```python
from build123d import *

# Parameters (mm, degrees)
SKETCH1_W           = 35
SKETCH1_H           = 35
BOSS_EXTRUDE1_DEPTH = 30


with BuildPart() as part:
    # Sketch1 → Boss-Extrude1 (new, symmetric)
    with BuildSketch(Plane(origin=(0, 0, 0), x_dir=(1, 0, 0), z_dir=(0, 1, 0))):
        Rectangle(SKETCH1_W, SKETCH1_H)
    extrude(amount=BOSS_EXTRUDE1_DEPTH, both=True)

    # Sketch3 → M5 Clearance Hole1 (revolve, cut)
    with BuildSketch(Plane(origin=(-12.5, 30, -12.5), x_dir=(0, 0, 1), z_dir=(1, 0, 0))):
        Polygon((0, 0), (0, 9.652366702), (2.75, 8), (2.75, 0), align=None)
    m5_clearance_hole1 = revolve(axis=Axis((-12.5, 36.35, -12.5), (0, -1, 0)), mode=Mode.SUBTRACT)

    # Mirror1: M5 Clearance Hole1 across plane
    add(m5_clearance_hole1.mirror(Plane(origin=(0, 0, 0), x_dir=(0, 0, 1), z_dir=(1, 0, 0))), mode=Mode.SUBTRACT)

    # Mirror2: M5 Clearance Hole1 across plane
    add(m5_clearance_hole1.mirror(Plane.XY), mode=Mode.SUBTRACT)

    # Mirror2 copy 1 sketch → Mirror2 copy 1 (revolve, cut)
    with BuildSketch(Plane(origin=(12.5, 30, 12.5), x_dir=(0, 0, -1), z_dir=(-1, 0, 0))):
        Polygon((0, 0), (0, 9.652366702), (2.75, 8), (2.75, 0), align=None)
    revolve(axis=Axis((12.5, 36.35, 12.5), (0, -1, 0)), mode=Mode.SUBTRACT)

    # Mirror3: M5 Clearance Hole1 across plane
    add(m5_clearance_hole1.mirror(Plane.ZX), mode=Mode.SUBTRACT)

    # Mirror3 copy 1 sketch → Mirror3 copy 1 (revolve, cut)
    with BuildSketch(Plane(origin=(12.5, -30, -12.5), x_dir=(0, 0, 1), z_dir=(-1, 0, 0))):
        Polygon((0, 0), (0, 9.652366702), (2.75, 8), (2.75, 0), align=None)
    revolve(axis=Axis((12.5, -36.35, -12.5), (0, 1, 0)), mode=Mode.SUBTRACT)

    # Mirror3 copy 2 sketch → Mirror3 copy 2 (revolve, cut)
    with BuildSketch(Plane(origin=(-12.5, -30, 12.5), x_dir=(0, 0, -1), z_dir=(1, 0, 0))):
        Polygon((0, 0), (0, 9.652366702), (2.75, 8), (2.75, 0), align=None)
    revolve(axis=Axis((-12.5, -36.35, 12.5), (0, 1, 0)), mode=Mode.SUBTRACT)

    # Mirror3 copy 3 sketch → Mirror3 copy 3 (revolve, cut)
    with BuildSketch(Plane(origin=(12.5, -30, 12.5), x_dir=(0, 0, -1), z_dir=(-1, 0, 0))):
        Polygon((0, 0), (0, -9.652366702), (2.75, -8), (2.75, 0), align=None)
    revolve(axis=Axis((12.5, -36.35, 12.5), (0, -1, 0)), mode=Mode.SUBTRACT)

    # Sketch8 → M4 Clearance Hole2 (revolve, cut)
    with BuildSketch(Plane(origin=(-17.5, 15, -12.5), x_dir=(0, 0, 1), z_dir=(0, 1, 0))):
        Polygon((0, 0), (0, 9.351936393), (2.25, 8), (2.25, 0), align=None)
    m4_clearance_hole2 = revolve(axis=Axis((-23.85, 15, -12.5), (1, 0, 0)), mode=Mode.SUBTRACT)

    # Mirror4: M4 Clearance Hole2 across plane
    add(m4_clearance_hole2.mirror(Plane.XY), mode=Mode.SUBTRACT)

    # Mirror5: M4 Clearance Hole2 across plane
    add(m4_clearance_hole2.mirror(Plane.ZX), mode=Mode.SUBTRACT)

    # Mirror5 copy 1 sketch → Mirror5 copy 1 (revolve, cut)
    with BuildSketch(Plane(origin=(-17.5, -15, 12.5), x_dir=(0, 0, -1), z_dir=(0, -1, 0))):
        Polygon((0, 0), (0, 9.351936393), (2.25, 8), (2.25, 0), align=None)
    revolve(axis=Axis((-23.85, -15, 12.5), (1, 0, 0)), mode=Mode.SUBTRACT)


solid = part.part
```
For this review, take the finished solid that the model builds, in its own axes (mm). A direction names the side the tool comes from. Coordinates: 2 decimals unless noted, no trailing zeros. Loops run counter-clockwise (first coordinate to the right, second up) from the corner with the lowest first, then second, coordinate; pieces in that order, holes last. Notation, with made-up numbers: (-24, 83.25) -> (27, 83.25) arc R17 cw to (27, 103.25) -> close; hole circle Ø2 at (16, -23.75). An arc over 180 degrees is marked (long way). Return JSON: item names as keys, results as strings. Group by question number.
(1) Tool access review of faces 1 (the cylindrical face through (13.33, -26.06, 9.88)), 2 (the cylindrical face through (-13.556, 16.369, 14.286)), 3 (the cylindrical face through (13.33, 26.06, 9.88)): name each direction out of +Z, -Z, +X, -X, +Y, -Y from which nothing blocks a thin tool from reaching the whole face with its end or side.
(2) Mouldability with a two-part tool opening along Z and no side actions: class faces 4 (the flat face through (0, 0, -17.5)), 5 (the flat face through (0, 0, 17.5)), 6 (the flat face through (0, -30, 0)), 7 (the conical face through (-12.643, 20.635, 12.044)) as pulls with the +Z half, pulls with the -Z half, needs draft (parallel to the pull), parting line crosses it, or undercut.
(3) For pin 1 Ø3.5 at (x, z) = (-12.5, -12.5) entering from -Y; pin 2 Ø5 at (x, z) = (12.5, 12.5) entering from +Y; pin 3 Ø3.5 at (x, z) = (-12.5, 12.5) entering from +Y, all flat-tipped, find the tip position at first contact; note any pin that passes through.
(4) To check wall thickness, follow L1, parallel to X at y = 23.5, z = 12.5; L2, parallel to Z at x = -15.75, y = 15. State the ranges of each line that lie inside material, in increasing order.
(5) Consider section A-A, the plane y = -24. Give the boundary of the cut face in (x, z).
Results below:
{
 "1": {"face 1": "-Y", "face 2": "-X", "face 3": "+Y"},
 "2": {"face 4": "pulls with the -Z half", "face 5": "pulls with the +Z half", "face 6": "needs draft", "face 7": "undercut"},
 "3": {"pin 1": "stops at y = -21.4", "pin 2": "stops at y = 21.85", "pin 3": "stops at y = 21.4"},
 "4": {"L1": "x = -17.5 to -15.25, -9.75 to 9.75, 15.25 to 17.5", "L2": "z = -17.5 to -14.75, -10.25 to 10.25, 14.75 to 17.5"},
 "5": {"outline": "(-17.5, -17.5) -> (17.5, -17.5) -> (17.5, 17.5) -> (-17.5, 17.5) -> close; hole circle Ø5.5 at (-12.5, -12.5); hole circle Ø5.5 at (-12.5, 12.5); hole circle Ø5.5 at (12.5, -12.5); hole circle Ø5.5 at (12.5, 12.5)"}
}
